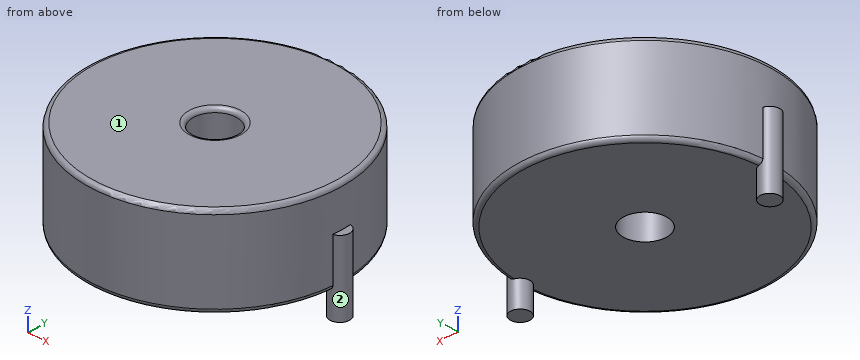
```python
from build123d import *

# Parameters (mm, degrees)
SKETCH001_R       = 1.15
PAD001_DEPTH      = 5.25
PAD001_DEPTH_BACK = 3.5
SKETCH_R          = 14.9
SKETCH_R_2        = 2.55
PAD_DEPTH         = 10.5
FILLET_R          = 0.5


with BuildPart() as pad001:
    # Sketch001 → Pad001 (new body, two sides)
    with BuildSketch(Plane.XY.offset(0.5)) as pad001_sk:
        Circle(SKETCH001_R)
        with Locations((29.3, 0)):
            Circle(SKETCH001_R)
    extrude(amount=PAD001_DEPTH)
    extrude(pad001_sk.sketch, amount=-PAD001_DEPTH_BACK)


with BuildPart() as obj1:
    # Sketch → Pad (new body)
    with BuildSketch(Plane.XY.offset(0.1)):
        with Locations((14.65, 0)):
            Circle(SKETCH_R)
        with Locations((14.65, 0)):
            Circle(SKETCH_R_2, mode=Mode.SUBTRACT)
    extrude(amount=PAD_DEPTH)

    # Fillet
    fillet_edges = [obj1.edges().sort_by_distance(p)[0] for p in [
        (12.1, 0, 10.6),
        (-0.25, 0, 10.6),
        (-0.25, 0, 0.1),
    ]]
    fillet(fillet_edges, radius=FILLET_R)

    # obj1: union Pad001
    add(pad001.part)


solid = obj1.part
```
Verification items for the finished model (mm, model axes). Face numbers are marked on the shaded views. A direction names the side the tool comes from. Coordinates: 2 decimals unless noted, no trailing zeros. Loops run counter-clockwise (first coordinate to the right, second up) from the corner with the lowest first, then second, coordinate; pieces in that order, holes last. Notation, with made-up numbers: (-20, 35.5) - (-3, 35.5) arc R32 cw to (-3, 61.5) - close; hole circle Ø9 at (4, 12.25). An arc over 180 degrees is marked (long way). Put each result on its own line as item: value.
Item 1: Section check D-D (z = 3.5). Enter the section's corners in (x, y).
Conclusion:
outline: (-0.21, -1.13) arc R14.9 ccw to (29.51, -1.13) arc R1.15 ccw to (29.51, 1.13) arc R14.9 ccw to (-0.21, 1.13) arc R1.15 ccw to start; hole circle Ø5.1 at (14.65, 0)
Item 2: Section check C-C (z = -0.5). Enter the section's corners in (x, y).
Conclusion:
outline: circle Ø2.3 at (0, 0); circle Ø2.3 at (29.3, 0)
Item 3: Section check B-B (x = 14.65). Enter the section's corners in (y, z).
Conclusion:
outline: (-14.9, 0.6) arc R0.5 ccw to (-14.4, 0.1) - (-2.55, 0.1) - (-2.55, 10.1) arc R0.5 ccw to (-3.05, 10.6) - (-14.4, 10.6) arc R0.5 ccw to (-14.9, 10.1) - close; (2.55, 0.1) - (14.4, 0.1) arc R0.5 ccw to (14.9, 0.6) - (14.9, 10.1) arc R0.5 ccw to (14.4, 10.6) - (3.05, 10.6) arc R0.5 ccw to (2.55, 10.1) - close
Item 4: Section check A-A (y = 0). Enter the section's corners in (x, z).
Conclusion:
outline: (-1.15, -3) - (1.15, -3) - (1.15, 0.1) - (12.1, 0.1) - (12.1, 10.1) arc R0.5 ccw to (11.6, 10.6) - (0.25, 10.6) arc R0.5 ccw to (-0.25, 10.1) - (-0.25, 5.75) - (-1.15, 5.75) - close; (17.2, 0.1) - (28.15, 0.1) - (28.15, -3) - (30.45, -3) - (30.45, 5.75) - (29.55, 5.75) - (29.55, 10.1) arc R0.5 ccw to (29.05, 10.6) - (17.7, 10.6) arc R0.5 ccw to (17.2, 10.1) - close
Item 5: Gauge pin test, flat ends, axial feed: pin 1 Ø1.5 at (x, z) = (21.5, 1.5) entering from -Y; pin 2 Ø1.5 at (x, z) = (9.5, 6) entering from +Y; pin 3 Ø14.5 at (x, y) = (12.5, 4.5) entering from -Z. Record the tip position at first contact, or that the pin passes through.
Conclusion:
pin 1: stops at y = -13.59
pin 2: stops at y = 14.24
pin 3: stops at z = 0.1
Item 6: Set-up check for the marked faces 1 and 2: record each of +Z, -Z, +X, -X, +Y, -Y from which the full face is reachable in a straight line by a thin tool's end or side.
Conclusion:
face 1: +Z, +X, -X, +Y, -Y
face 2: -Z
Item 7: Scan lines: line 1 along Y through (x, z) = (14.65, 5.25); line 2 along Z through (x, y) = (23.5, 1.75); line 3 along Y through (x, z) = (2, 3). Record each from-to range of solid material in increasing order.
Conclusion:
line 1: y = -14.9 to -2.55, 2.55 to 14.9
line 2: z = 0.1 to 10.6
line 3: y = -7.87 to 7.87
